Geometry: final body of the model. Coordinates: model frame, mm. A direction names the side the tool comes from. Give positions to 0.01 mm unless a question says otherwise; leave off trailing zeros. Loops run counter-clockwise (first coordinate to the right, second up) from the corner with the lowest first, then second, coordinate; pieces in that order, holes last. Notation, with made-up numbers: (38.5, -28.75) - (43.5, -28.75) arc R22 cw to (43.5, 1.25) - close; hole circle Ø8 at (70.25, 25.25). An arc over 180 degrees is marked (long way). Use one line per item in the form item = value.
```python
from build123d import *

# Parameters (mm, degrees)
SKETCH1_W           = 20
SKETCH1_H           = 50
BOSS_EXTRUDE1_DEPTH = 70
SKETCH2_R           = 1.5
SKETCH2_R_2         = 11.5
CUT_EXTRUDE2_DEPTH  = 60
SKETCH4_W           = 34
SKETCH4_H           = 12
CUT_EXTRUDE3_DEPTH  = 60
SKETCH8_R           = 2
CUT_EXTRUDE5_DEPTH  = 15
SKETCH9_W           = 42
SKETCH9_H           = 42
CUT_EXTRUDE6_DEPTH  = 8
CUT_EXTRUDE8_DEPTH  = 30
SKETCH17_R          = 3.5
CUT_EXTRUDE13_DEPTH = 9.18109305
SKETCH18_R          = 1.5
CUT_EXTRUDE14_DEPTH = 7
FILLET1_R           = 2
FILLET2_R           = 2
FILLET3_R           = 2
FILLET4_R           = 2
SKETCH19_W          = 5
SKETCH19_H          = 42
BOSS_EXTRUDE2_DEPTH = 26
FILLET6_R           = 2


with BuildPart() as part:
    # Sketch1 → Boss-Extrude1 (new body)
    with BuildSketch(Plane(origin=(0, 0, 0), x_dir=(1, 0, 0), z_dir=(0, 1, 0))):
        with Locations((-10, -25)):
            Rectangle(SKETCH1_W, SKETCH1_H)
    extrude(amount=BOSS_EXTRUDE1_DEPTH)

    # Sketch2 → Cut-Extrude2 (cut)
    with BuildSketch(Plane(origin=(0, 0, 0), x_dir=(0, 0, -1), z_dir=(1, 0, 0))):
        with Locations((-8.5, 61)):
            Circle(SKETCH2_R)
        with Locations((-24, 45.5)):
            Circle(SKETCH2_R_2)
        with Locations((-8.5, 30)):
            Circle(SKETCH2_R)
        with Locations((-39.5, 30)):
            Circle(SKETCH2_R)
        with Locations((-39.5, 61)):
            Circle(SKETCH2_R)
    extrude(amount=-CUT_EXTRUDE2_DEPTH, mode=Mode.SUBTRACT)

    # Sketch4 → Cut-Extrude3 (cut)
    with BuildSketch(Plane(origin=(0, 0, 0), x_dir=(0, 0, -1), z_dir=(1, 0, 0))):
        with Locations((-33, 6)):
            Rectangle(SKETCH4_W, SKETCH4_H)
    extrude(amount=-CUT_EXTRUDE3_DEPTH, mode=Mode.SUBTRACT)

    # Sketch8 → Cut-Extrude5 (cut)
    with BuildSketch(Plane(origin=(0, 0, 0), x_dir=(-1, 0, 0), z_dir=(0, 0, -1))):
        with Locations((15, 6)):
            Circle(SKETCH8_R)
        with Locations((5, 6)):
            Circle(SKETCH8_R)
    extrude(amount=-CUT_EXTRUDE5_DEPTH, mode=Mode.SUBTRACT)

    # Sketch9 → Cut-Extrude6 (cut)
    with BuildSketch(Plane(origin=(0, 0, 0), x_dir=(0, 0, -1), z_dir=(1, 0, 0))):
        with Locations((-24, 45.5)):
            Rectangle(SKETCH9_W, SKETCH9_H)
    extrude(amount=-CUT_EXTRUDE6_DEPTH, mode=Mode.SUBTRACT)

    # Sketch11 → Cut-Extrude8 (cut)
    with BuildSketch(Plane(origin=(0, 0, 0), x_dir=(0, 0, -1), z_dir=(1, 0, 0))):
        Polygon((-10, 0), (0, 0), (0, 12), align=None)
    extrude(amount=-CUT_EXTRUDE8_DEPTH, mode=Mode.SUBTRACT)

    # Sketch17 → Cut-Extrude13 (cut)
    with BuildSketch(Plane(origin=(0, 0, 0), x_dir=(-1, 0, 0), z_dir=(0, 0, -1))):
        with Locations((15, 6)):
            Circle(SKETCH17_R)
        with Locations((5, 6)):
            Circle(SKETCH17_R)
    extrude(amount=-CUT_EXTRUDE13_DEPTH, mode=Mode.SUBTRACT)

    # Sketch18 → Cut-Extrude14 (cut)
    with BuildSketch(Plane.ZY.offset(20)):
        with Locations((46, 20)):
            Circle(SKETCH18_R)
        with Locations((39, 20)):
            Circle(SKETCH18_R)
    extrude(amount=-CUT_EXTRUDE14_DEPTH, mode=Mode.SUBTRACT)

    # Fillet1
    fillet1_edges = [part.edges().sort_by_distance(p)[0] for p in [
        (-20, 41, 0),
    ]]
    fillet(fillet1_edges, radius=FILLET1_R)

    # Fillet2
    fillet2_edges = [part.edges().sort_by_distance(p)[0] for p in [
        (-20, 70, 26),
        (-19.414213562, 70, 0.585786438),
        (-9, 70, 0),
    ]]
    fillet(fillet2_edges, radius=FILLET2_R)

    # Fillet3
    fillet3_edges = [part.edges().sort_by_distance(p)[0] for p in [
        (0, 40, 0),
        (0, 69.414213562, 0.585786438),
        (0, 70, 26),
    ]]
    fillet(fillet3_edges, radius=FILLET3_R)

    # Fillet4
    fillet4_edges = [part.edges().sort_by_distance(p)[0] for p in [
        (-10, 0, 10),
    ]]
    fillet(fillet4_edges, radius=FILLET4_R)

    # Sketch19 → Boss-Extrude2 (add)
    with BuildSketch(Plane(origin=(0, 0, 0), x_dir=(0, 0, -1), z_dir=(1, 0, 0))):
        with Locations((-47.5, 45.5)):
            Rectangle(SKETCH19_W, SKETCH19_H)
    extrude(amount=BOSS_EXTRUDE2_DEPTH)

    # Fillet6
    fillet6_edges = [part.edges().sort_by_distance(p)[0] for p in [
        (13, 66.5, 50),
        (13, 24.5, 50),
        (26, 45.5, 50),
    ]]
    fillet(fillet6_edges, radius=FILLET6_R)


solid = part.part
```
(1) Cut plane C-C (y = 52). Return the cut outline in (x, z), plus the area to 3 significant figures.
Solution:
outline = (-20, 2) arc R2 ccw to (-18, 0) - (-2, 0) arc R2 ccw to (0, 2) - (0, 3) - (-8, 3) - (-8, 14.51) - (-20, 14.51) - close; (-20, 33.49) - (-8, 33.49) - (-8, 45) - (26, 45) - (26, 48) arc R2 ccw to (24, 50) - (-20, 50) - close
area = 564 mm2
(2) Pull-direction query (Y, two-part tool) for faces 1 (the face through (-4.54, 9.47, 6.34)), 2 (the face through (-9.89, 69.4, 0.57)), 3 (the face through (25.4, 45.79, 49.43)); classes: released by +Y, released by -Y, zero draft, split by the parting line, or undercut.
Solution:
face_1 = undercut
face_2 = released by +Y
face_3 = zero draft
(3) Cut plane D-D (x = -15). Return the cut outline in (y, z).
Solution:
outline = (0, 10.94) arc R2 ccw to (0.72, 9.4) - (2.5, 7.92) - (2.5, 9.18) - (4, 9.18) - (4, 15) - (8, 15) - (8, 9.18) - (9.5, 9.18) - (9.5, 2.08) - (12, 0) - (68, 0) arc R2 ccw to (70, 2) - (70, 50) - (12, 50) - (12, 16) - (0, 16) - close; hole circle Ø3 at (20, 39); hole circle Ø3 at (20, 46); hole circle Ø3 at (30, 8.5); hole circle Ø3 at (30, 39.5); hole circle Ø23 at (45.5, 24); hole circle Ø3 at (61, 8.5); hole circle Ø3 at (61, 39.5)
(4) Access query for faces 4 (the face through (13.18, 65.9, 49.43)), 5 (the face through (-3, 6, 12)), 6 (the face through (-4, 45, 3)), 7 (the face through (13.18, 25.1, 49.43)), 8 (the face through (-16.55, 20.07, 44.5)). Directions: +Z, -Z, +X, -X, +Y, -Y. A direction counts if a zero-diameter tool reaches every point of the face in a straight line with its end or side. Return the directions, or none.
Solution:
face_4 = +Z, +X, +Y
face_5 = -Z
face_6 = +X
face_7 = +Z, +X, -Y
face_8 = -X
(5) Cut plane B-B (z = 24). Return the cut outline in (x, y), plus the area to 3 significant figures.
Solution:
outline = (-20, 12) - (0, 12) - (0, 24.5) - (-8, 24.5) - (-8, 34) - (-20, 34) - close; (-20, 57) - (-8, 57) - (-8, 66.5) - (0, 66.5) - (0, 68) arc R2 ccw to (-2, 70) - (-18, 70) arc R2 ccw to (-20, 68) - close
area = 546 mm2
(6) Material intervals for L1, parallel to X at y = 6, z = 5.5; L2, parallel to X at y = 25, z = 38; L3, parallel to Y at x = -15, z = 11, sorted ascending. Write a range as from..to.
Solution:
L1 = -20..-18.5, -11.5..-8.5, -1.5..0
L2 = -20..-8
L3 = 0..4, 8..70
(7) Pin query (flat end, axial travel): P1, Ø1.5, axis at y = 20.5, z = 46, coming from the -X side; P2, Ø14.5, axis at y = 29, z = 34, coming from the +X side; P3, Ø8, axis at x = -5, y = 6, coming from the +Z side. Return the tip coordinate at first contact, or that it passes through.
Solution:
P1 = -13
P2 = 0
P3 = 16
(8) Cut plane A-A (y = 61). Return the cut outline in (x, z), plus the area to 3 significant figures.
Solution:
outline = (-20, 2) arc R2 ccw to (-18, 0) - (-2, 0) arc R2 ccw to (0, 2) - (0, 3) - (-8, 3) - (-8, 7) - (-20, 7) - close; (-20, 10) - (-8, 10) - (-8, 38) - (-20, 38) - close; (-20, 41) - (-8, 41) - (-8, 45) - (26, 45) - (26, 48) arc R2 ccw to (24, 50) - (-20, 50) - close
area = 719 mm2
